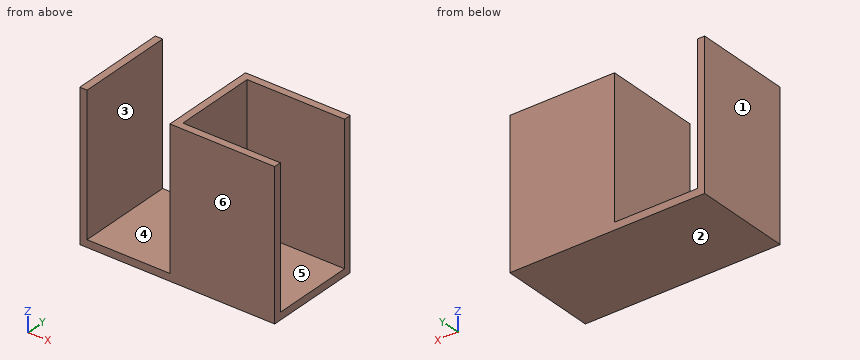
from build123d import *

# Parameters (mm, degrees)
F0_W     = 20
F0_H     = 30
F1_DEPTH = 20
F3_W     = 17
F3_H     = 28.5
F4_DEPTH = 30


with BuildPart() as f1:
    # F0 (on Front) → F1 (new body)
    with BuildSketch(Plane.XZ):
        Polygon((-18.5, 30), (-20, 30), (-20, 0), (0, 0), (0, 30), (-1.5, 30), (-1.5, 1.5), (-18.5, 1.5), align=None)
        with Locations((10, 15)):
            Rectangle(F0_W, F0_H)
    extrude(amount=F1_DEPTH)

    # F3 (on offset) → F4 (cut)
    with BuildSketch(Plane.YZ.offset(30)):
        with Locations((-10, 15.75)):
            Rectangle(F3_W, F3_H)
    extrude(amount=-F4_DEPTH, mode=Mode.SUBTRACT)


solid = f1.part
Part model, mm, in its own coordinate system. Face numbers are marked on the shaded views. A direction names the side the tool comes from. Round coordinates to 2 decimals unless told otherwise and drop trailing zeros. Write each loop counter-clockwise with the first axis right and the second up, starting at its lowest first coordinate (ties: lowest second). Pieces come first, ordered by that corner, then holes. Notation, with made-up numbers: M 80.25,-24 L 121.25,-24 A14 ccw 121.25,-13 Z; hole C 12.25,87 d10. An arc over 180 degrees is marked long. Return JSON: item names as keys, results as strings. Group by question number.
(1) Which spindle directions (+Z, -Z, +X, -X, +Y, -Y) get a long thin tool onto all of the face, cutting with end or side? Do the marked faces 4, 5 and 6. Say none if no direction does.
(2) Pin check, flat tips, straight feed: pin 1 Ø8 at (y, z) = (-2.5, 19) entering from +X; pin 2 Ø5 at (x, y) = (14, -10) entering from +Z; pin 3 Ø8.5 at (y, z) = (-12.5, 10.5) entering from +X. Stop position of each tip, or through.
(3) Drill centre lines: probe 1 along X at (y, z) = (-5.75, 28.5); probe 2 along Z at (x, y) = (-13, -10). Where is each one in solid material? Low to high.
(4) Two-plate mould, pull along X, no slides. Class the marked faces 1, 2 and 3: +X half, -X half, draft (parallel to the pull), parting line (faces both ways), or undercut.
(5) Saw through at D-D on y = -1. Write the cut outline in (x, z), then the cut area to 4 significant figures.
(6) Saw through at A-A on z = 8.75. Write the cut outline in (x, y), then the cut area to 3 significant figures.
(7) Saw through at B-B on y = -8. Write the cut outline in (x, z).
(8) Saw through at C-C on x = 5. Write the cut outline in (y, z).
Returned:
{
 "1": {"face 4": "+Z, +Y, -Y", "face 5": "+Z, +X", "face 6": "+Z, -Z, +X, -X, -Y"},
 "2": {"pin 1": "x = 20", "pin 2": "z = 1.5", "pin 3": "x = 0"},
 "3": {"probe 1": "-20 to -18.5, -1.5 to 0", "probe 2": "0 to 1.5"},
 "4": {"face 1": "-X half", "face 2": "draft", "face 3": "undercut"},
 "5": {"outline": "M -20,0 L 20,0 L 20,30 L -1.5,30 L -1.5,1.5 L -18.5,1.5 L -18.5,30 L -20,30 Z", "area": "715.5 mm²"},
 "6": {"outline": "M -20,-20 L -18.5,-20 L -18.5,0 L -20,0 Z; M -1.5,-20 L 20,-20 L 20,-18.5 L 0,-18.5 L 0,-1.5 L 20,-1.5 L 20,0 L -1.5,0 Z", "area": "120 mm²"},
 "7": {"outline": "M -20,0 L 20,0 L 20,1.5 L 0,1.5 L 0,30 L -1.5,30 L -1.5,1.5 L -18.5,1.5 L -18.5,30 L -20,30 Z"},
 "8": {"outline": "M -20,0 L 0,0 L 0,30 L -1.5,30 L -1.5,1.5 L -18.5,1.5 L -18.5,30 L -20,30 Z"}
}
